Verification items for the finished model (mm, model axes). Face numbers are marked on the shaded views. A direction names the side the tool comes from. Round coordinates to 2 decimals unless told otherwise and drop trailing zeros. Order: outer loops, then holes, each group sorted by start corner. A loop starts at its lowest first (then second) coordinate and runs counter-clockwise, first axis right, second up. Notation, with made-up numbers: M 27,27 L 78,27 A7 ccw 78,37 Z; hole C 12.25,65 d2. An arc over 180 degrees is marked long. Use CSV: the item, a comma, the result in double quotes. Start each with the question number.
Q1. Mould release check, pull along Z, two halves, no side actions. Record for the marked faces 1, 2 and 3: +Z half, -Z half, draft (parallel to the pull), parting line (faces both ways), or undercut.
Q2. Set-up check for the marked faces 4, 5 and 6: record each of +Z, -Z, +X, -X, +Y, -Y from which the full face is reachable in a straight line by a thin tool's end or side.
Q3. Sectioned sample at B-B (z = 0). Enter the section's corners in (x, y), and give its area (3 significant figures).
Q4. Sectioned sample at D-D (x = 3). Enter the section's corners in (y, z).
Q5. Sectioned sample at C-C (y = -3). Enter the section's corners in (x, z).
Q6. Scan lines: line 1 (X direction, y = 15, z = 0); line 2 (Z direction, x = 0, y = 1.5); line 3 (Y direction, x = -8, z = 0.25). Record each from-to range of solid material in increasing order.
Q7. Gauge pin test, flat ends, axial feed: pin 1 Ø5 at (x, y) = (6, -2.5) entering from -Z; pin 2 Ø3.5 at (x, y) = (-6, -8.5) entering from +Z; pin 3 Ø1.3 at (x, y) = (-6, -10.5) entering from -Z; pin 4 Ø4.5 at (x, z) = (0, 0) entering from -Y. Record the tip position at first contact, or that the pin passes through.
Q8. Sectioned sample at A-A (x = 0). Enter the section's corners in (y, z), and give its area (3 significant figures).
Autodesk Inventor part; units mm, degrees
ref_plane "YZ Plane" through (0, 0, 0) normal (1, 0, 0) x (0, 1, 0)
ref_plane "XZ Plane" through (0, 0, 0) normal (0, 1, 0) x (-1, 0, 0)
ref_plane "XY Plane" through (0, 0, 0) normal (0, 0, 1) x (1, 0, 0)
sketch "Sketch1" plane through (0, 0, 0) normal (0, 0, 1) x (1, 0, 0)
  line L0 (0, 17.5) -> (9, 17.5)
  line L1 (9, 17.5) -> (9, -17.5)
  line L2 (9, -17.5) -> (0, -17.5)
  line L3 (0, -17.5) -> (0, 17.5)
  line L4 (0, 7.5) -> (2.45, 7.5)
  line L5 (2.45, 7.5) -> (2.45, 17.5)
  line L6 (2.45, 17.5) -> (0, 17.5)
  line L7 (0, 17.5) -> (0, 7.5)
  line L8 (0, 7.5) -> (5, 7.5)
  line L9 (5, 7.5) -> (5, -17.5)
  line L10 (5, -17.5) -> (0, -17.5)
  line L11 (0, -17.5) -> (0, 7.5)
  point P0 (0, 0)
  dimension "d0" = 9
  dimension "d1" = 35
  dimension "d2" = 17.5
  dimension "d3" = 10
  dimension "d4" = 2.45
  dimension "d5" = 5
revolve "Revolution1" add sketch "Sketch1" angle 360 about axis through (0, -17.5, 0) along (0, 1, 0) contours L0 L1 L2 L9 L8 L5
sketch "Sketch2" plane through (0, 0, 0) normal (1, 0, 0) x (0, 1, 0)
  line L0 (-17.5, 5) -> (-17.5, -5)
  line L1 (2.5, 3) -> (-17.5, 3)
  line L2 (-17.5, 3) -> (-17.5, -3)
  line L3 (-17.5, -3) -> (2.5, -3)
  line L4 (2.5, -3) -> (2.5, 3)
  line L5 (-17.5, 5) -> (7.5, 5)
  line L6 (-17.5, -5) -> (7.5, -5)
  line L7 (7.5, 5) -> (7.5, -5)
  point P0 (2.5, 0)
  dimension "d7" = 2
  dimension "d8" = 2
  dimension "d11" = 5
extrude "Extrusion1" cut sketch "Sketch2" along normal through all both and the other way through all contours L1 L4 L3 L0
properties part number "mini fidget foot"
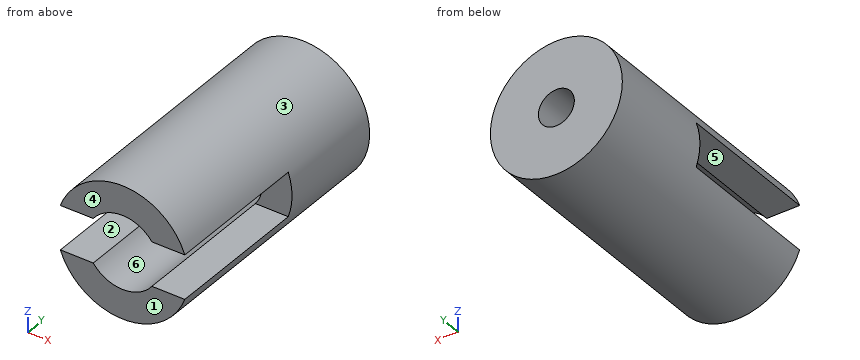
Verdict:
1,face 1,"draft"
1,face 2,"undercut"
1,face 3,"parting line"
2,face 4,"+Z, -Z, +X, -X, -Y"
2,face 5,"+X, -X, -Y"
2,face 6,"-Y"
3,outline,"M -9,2.5 L -5,2.5 L -5,7.5 L -2.45,7.5 L -2.45,17.5 L -9,17.5 Z; M 2.45,7.5 L 5,7.5 L 5,2.5 L 9,2.5 L 9,17.5 L 2.45,17.5 Z"
3,area,"171 mm²"
4,outline,"M -17.5,-8.49 L 17.5,-8.49 L 17.5,8.49 L -17.5,8.49 L -17.5,4 L 7.5,4 L 7.5,-4 L -17.5,-4 Z"
5,outline,"M -8.49,-3 A9 ccw 8.49,-3 L 4,-3 A5 cw -4,-3 Z; M -8.49,3 L -4,3 A5 cw 4,3 L 8.49,3 A9 ccw Z"
6,line 1,"x = -9 to -2.45, 2.45 to 9"
6,line 2,"z = -9 to -5, 5 to 9"
6,line 3,"y = 2.5 to 17.5"
7,pin 1,"stops at z = -8.29"
7,pin 2,"stops at z = 7.93"
7,pin 3,"stops at z = -7.24"
7,pin 4,"passes through"
8,outline,"M -17.5,-9 L 17.5,-9 L 17.5,-2.45 L 7.5,-2.45 L 7.5,-5 L -17.5,-5 Z; M -17.5,5 L 7.5,5 L 7.5,2.45 L 17.5,2.45 L 17.5,9 L -17.5,9 Z"
8,area,"331 mm²"
